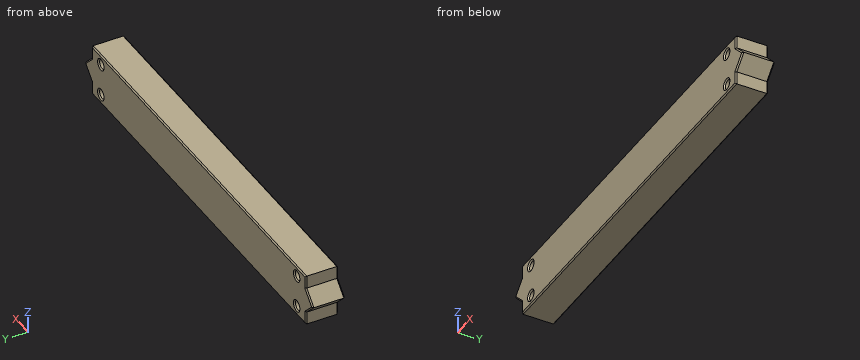
```python
from build123d import *

# Parameters (mm, degrees)
SKETCH1_R           = 1.8
BOSS_EXTRUDE1_DEPTH = 12.7
CHAMFER1_SIZE       = 0.5


with BuildPart() as part:
    # Sketch1 → Boss-Extrude1 (new body)
    with BuildSketch(Plane(origin=(0, 0, 0), x_dir=(1, 0, 0), z_dir=(0, 1, 0))):
        Polygon((-76.2, 5.08), (-81.28, 0), (-76.2, -5.08), (-76.2, -10.16), (76.2, -10.16), (76.2, -5.08), (81.28, 0), (76.2, 5.08), (76.2, 10.16), (-76.2, 10.16), align=None)
        with Locations(Location((-69.85, 6.35, 0), (0, 0, 270))):
            Circle(SKETCH1_R, mode=Mode.SUBTRACT)
        with Locations(Location((-69.85, -6.35, 0), (0, 0, 90))):
            Circle(SKETCH1_R, mode=Mode.SUBTRACT)
        with Locations(Location((69.85, -6.35, 0), (0, 0, 270))):
            Circle(SKETCH1_R, mode=Mode.SUBTRACT)
        with Locations(Location((69.85, 6.35, 0), (0, 0, 90))):
            Circle(SKETCH1_R, mode=Mode.SUBTRACT)
    extrude(amount=BOSS_EXTRUDE1_DEPTH)

    # Chamfer1
    chamfer1_edges = [part.edges().sort_by_distance(p)[0] for p in [
        (0, 0, 10.16),
        (-76.2, 0, 7.62),
        (-78.74, 0, 2.54),
        (-78.74, 0, -2.54),
        (-76.2, 0, -7.62),
        (0, 0, -10.16),
        (76.2, 0, -7.62),
        (78.74, 12.7, -2.54),
        (78.74, 0, -2.54),
        (78.74, 0, 2.54),
        (76.2, 0, 7.62),
        (76.2, 12.7, -7.62),
        (0, 12.7, -10.16),
        (-76.2, 12.7, -7.62),
        (-69.85, 0, -8.15),
        (-69.85, 12.7, -8.15),
        (-78.74, 12.7, -2.54),
        (-69.85, 0, 8.15),
        (-69.85, 12.7, 8.15),
        (-78.74, 12.7, 2.54),
        (69.85, 0, 4.55),
        (69.85, 12.7, 4.55),
        (-76.2, 12.7, 7.62),
        (69.85, 0, -4.55),
        (69.85, 12.7, -4.55),
        (0, 12.7, 10.16),
        (76.2, 12.7, 7.62),
        (78.74, 12.7, 2.54),
    ]]
    chamfer(chamfer1_edges, length=CHAMFER1_SIZE)


solid = part.part
```
Check sheet for the modelled part. Datum: model origin and axes. Units: mm. Give positions to 0.01 mm unless a question says otherwise; leave off trailing zeros. Write each loop counter-clockwise with the first axis right and the second up, starting at its lowest first coordinate (ties: lowest second). Pieces come first, ordered by that corner, then holes.
Item 1: Cross-section at B-B (y = 4). Enter the section's corners in (x, z).
Item 2: Scan lines: L1, parallel to X at y = 9.5, z = 6.35; L2, parallel to Z at x = 69.85, y = 9.25; L3, parallel to X at y = 4, z = -4.75. Record each from-to range of solid material in increasing order.
Item 3: Gauge pin test, flat ends, axial feed: pin 1 (5 mm diameter, centred on x = 60.5, z = 3.5, fed in from -Y); pin 2 (5.5 mm diameter, centred on y = 9, z = 8, fed in from +X); pin 3 (5.5 mm diameter, centred on y = 4, z = -9, fed in from -X); pin 4 (2 mm diameter, centred on x = -69.85, z = -6.35, fed in from -Y). Record the tip position at first contact, or that the pin passes through.
Item 4: Cross-section at A-A (x = 69.85). Enter the section's corners in (y, z), and give its area (3 significant figures).
Report:
1. outline: (-81.28, 0) - (-76.2, -5.08) - (-76.2, -10.16) - (76.2, -10.16) - (76.2, -5.08) - (81.28, 0) - (76.2, 5.08) - (76.2, 10.16) - (-76.2, 10.16) - (-76.2, 5.08) - close; hole circle Ø3.6 at (-69.85, -6.35); hole circle Ø3.6 at (-69.85, 6.35); hole circle Ø3.6 at (69.85, -6.35); hole circle Ø3.6 at (69.85, 6.35)
2. L1: x = -76.2 to -71.65, -68.05 to 68.05, 71.65 to 76.2
2. L2: z = -10.16 to -8.15, -4.55 to 4.55, 8.15 to 10.16
2. L3: x = -76.53 to -70.67, -69.03 to 69.03, 70.67 to 76.53
3. pin 1: stops at y = 0
3. pin 2: stops at x = 76.2
3. pin 3: stops at x = -76.2
3. pin 4: passes through
4. outline: (0, -9.66) - (0.5, -10.16) - (12.2, -10.16) - (12.7, -9.66) - (12.7, -8.65) - (12.2, -8.15) - (0.5, -8.15) - (0, -8.65) - close; (0, -4.05) - (0.5, -4.55) - (12.2, -4.55) - (12.7, -4.05) - (12.7, 4.05) - (12.2, 4.55) - (0.5, 4.55) - (0, 4.05) - close; (0, 8.65) - (0.5, 8.15) - (12.2, 8.15) - (12.7, 8.65) - (12.7, 9.66) - (12.2, 10.16) - (0.5, 10.16) - (0, 9.66) - close
4. area: 165 mm2
